For this review, take the finished solid that the model builds, in its own axes (mm). A direction names the side the tool comes from. Give positions to 0.01 mm unless a question says otherwise; leave off trailing zeros. Loops run counter-clockwise (first coordinate to the right, second up) from the corner with the lowest first, then second, coordinate; pieces in that order, holes last. Notation, with made-up numbers: M 16.5,-7.75 L 47.5,-7.75 A23 cw 47.5,3.25 Z; hole C -21,73 d11. An arc over 180 degrees is marked long. Use CSV: the item, a comma, the result in double quotes. Start each with the question number.
1. Insertion check: P1, Ø1.2, axis at y = 12.5, z = 1, coming from the +X side; P2, Ø10, axis at x = -1, y = 17, coming from the +Z side; P3, Ø2.5, axis at x = -5, z = 1, coming from the +Y side. Each pin has a flat end and moves straight along its axis. Give the tip position at first contact, or say it passes through.
2. Tool access review of faces 4 (the face through (14.507, 6.536, 1.325)), 5 (the face through (14, 10, 0)): name each direction out of +Z, -Z, +X, -X, +Y, -Y from which nothing blocks a thin tool from reaching the whole face with its end or side.
3. Take a section at B-B, the plane y = 8. Write out the cut boundary in (x, z).
4. Take a section at D-D, the plane x = -10. Write out the cut boundary in (y, z).
5. Take a section at C-C, the plane z = -1.5. Write out the cut boundary in (x, y), and give its area (3 significant figures).
6. The part is to be moulded in two halves that separate along Z. For faces 1 (the face through (-14.507, 15.916, 2.535)), 2 (the face through (8.536, 0.986, 1.325)), 3 (the face through (0, 0, -1)), say which applies: pulls with the +Z half, pulls with the -Z half, needs draft (parallel to the pull), parting line crosses it, or undercut.
7. Take a section at A-A, the plane x = 5. Write out the cut boundary in (y, z), and give its area (3 significant figures).
8. To check wall thickness, follow line 1 (X direction, y = 1.4, z = 1); line 2 (X direction, y = 3, z = 4.5); line 3 (Y direction, x = 14.7, z = 1). State the ranges of each line that lie inside material, in increasing order. Write a range as [from, to].
from build123d import *

# Parameters (mm, degrees)
SKETCH1_W           = 30
SKETCH1_H           = 10
BOSS_EXTRUDE1_DEPTH = 2
SKETCH2_W           = 30
SKETCH2_H           = 2
BOSS_EXTRUDE2_DEPTH = 20
BOSS_EXTRUDE3_DEPTH = 1
BOSS_EXTRUDE4_START = -30
BOSS_EXTRUDE4_DEPTH = 1
SKETCH4_R           = 1.5
SKETCH4_R_2         = 1
CUT_EXTRUDE1_DEPTH  = 11
SKETCH5_R           = 1.5
SKETCH5_R_2         = 1
CUT_EXTRUDE2_DEPTH  = 41


with BuildPart() as part:
    # Sketch1 → Boss-Extrude1 (new body)
    with BuildSketch(Plane(origin=(0, 0, 0), x_dir=(1, 0, 0), z_dir=(0, 1, 0))):
        Rectangle(SKETCH1_W, SKETCH1_H)
    extrude(amount=BOSS_EXTRUDE1_DEPTH)

    # Sketch2 → Boss-Extrude2 (add)
    with BuildSketch(Plane(origin=(0, 2, 0), x_dir=(1, 0, 0), z_dir=(0, 1, 0))):
        with Locations((0, 4)):
            Rectangle(SKETCH2_W, SKETCH2_H)
    extrude(amount=BOSS_EXTRUDE2_DEPTH)

    # Sketch3 → Boss-Extrude3 (add)
    with BuildSketch(Plane(origin=(15, 0, 0), x_dir=(0, 0, -1), z_dir=(1, 0, 0))):
        Polygon((-5, 2), (-5, 10), (0, 22), (3, 22), (3, 2), align=None)
    extrude(amount=-BOSS_EXTRUDE3_DEPTH)

    # Sketch3<2> → Boss-Extrude4 (add)
    with BuildSketch(Plane(origin=(15, 0, 0), x_dir=(0, 0, -1), z_dir=(1, 0, 0)).offset(BOSS_EXTRUDE4_START)):
        Polygon((-5, 2), (-5, 10), (0, 22), (3, 22), (3, 2), align=None)
    extrude(amount=BOSS_EXTRUDE4_DEPTH)

    # Sketch4 → Cut-Extrude1 (cut)
    with BuildSketch(Plane.XZ):
        with Locations(Location((0, 1, 0), (0, 0, 270))):
            Circle(SKETCH4_R)
        with Locations(Location((5, 1, 0), (0, 0, 270))):
            Circle(SKETCH4_R_2)
        with Locations(Location((-5, 1, 0), (0, 0, 270))):
            Circle(SKETCH4_R_2)
        with Locations(Location((10, 1, 0), (0, 0, 270))):
            Circle(SKETCH4_R)
        with Locations(Location((-10, 1, 0), (0, 0, 270))):
            Circle(SKETCH4_R)
    extrude(amount=-CUT_EXTRUDE1_DEPTH, mode=Mode.SUBTRACT)

    # Sketch5 → Cut-Extrude2 (cut)
    with BuildSketch(Plane(origin=(15, 0, 0), x_dir=(0, 0, -1), z_dir=(1, 0, 0))):
        with Locations((-1, 8)):
            Circle(SKETCH5_R)
        with Locations((-1, 12.5)):
            Circle(SKETCH5_R_2)
    extrude(amount=-CUT_EXTRUDE2_DEPTH, mode=Mode.SUBTRACT)


solid = part.part
Result set:
1,P1,"through"
1,P2,"z = -3"
1,P3,"y = 2"
2,face 4,"+X, -X"
2,face 5,"+Z, +Y"
3,outline,"M -15,-5 L 15,-5 L 15,-0.5 L 14,-0.5 L 14,-3 L -14,-3 L -14,-0.5 L -15,-0.5 Z; M -15,2.5 L -14,2.5 L -14,5 L -15,5 Z; M 14,2.5 L 15,2.5 L 15,5 L 14,5 Z"
4,outline,"M 0,-5 L 22,-5 L 22,-3 L 2,-3 L 2,-0.5 L 0,-0.5 Z; M 0,2.5 L 2,2.5 L 2,5 L 0,5 Z"
5,outline,"M -15,0 L 15,0 L 15,22 L 14,22 L 14,2 L -14,2 L -14,22 L -15,22 Z"
5,area,"100 mm2"
6,face 1,"pulls with the +Z half"
6,face 2,"undercut"
6,face 3,"needs draft"
7,outline,"M 0,-5 L 22,-5 L 22,-3 L 2,-3 L 2,0 L 0,0 Z; M 0,2 L 2,2 L 2,5 L 0,5 Z"
7,area,"56.0 mm2"
8,line 1,"[-15, -11.5], [-8.5, -6], [-4, -1.5], [1.5, 4], [6, 8.5], [11.5, 15]"
8,line 2,"[-15, -14], [14, 15]"
8,line 3,"[0, 6.5], [9.5, 11.5], [13.5, 19.6]"
